Work out the finished part from the listing and answer in its coordinate system (mm). A direction names the side the tool comes from. Give positions to 0.01 mm unless a question says otherwise; leave off trailing zeros. Order: outer loops, then holes, each group sorted by start corner. A loop starts at its lowest first (then second) coordinate and runs counter-clockwise, first axis right, second up. Notation, with made-up numbers: (67.25, 52.5) -> (77.25, 52.5) arc R22 cw to (77.25, 80.5) -> close; hole circle Ø5 at (54.25, 74). An arc over 180 degrees is marked (long way). Use a Markdown table: item, result. Add a question column.
Autodesk Inventor part; units mm, degrees
ref_plane "YZ Plane" through (0, 0, 0) normal (1, 0, 0) x (0, 1, 0)
ref_plane "XZ Plane" through (0, 0, 0) normal (0, 1, 0) x (-1, 0, 0)
ref_plane "XY Plane" through (0, 0, 0) normal (0, 0, 1) x (1, 0, 0)
sketch "Sketch9" plane through (0, 0, 0) normal (0, 1, 0) x (-1, 0, 0)
  line L0 (15, 15) -> (-15, 15)
  line L1 (-15, 15) -> (-15, -15)
  line L2 (-15, -15) -> (15, -15)
  line L3 (15, -15) -> (15, 15)
  line L4 (15, 15) -> (-15, -15) construction
  line L5 (-15, 15) -> (15, -15) construction
  line L6 (-13, 13) -> (13, 13)
  line L7 (13, 13) -> (13, -13)
  line L8 (13, -13) -> (-13, -13)
  line L9 (-13, -13) -> (-13, 13)
  point P0 (0, 0)
  dimension "d172" = 30
  dimension "d173" = 30
  dimension "d174" = 2
extrude "Extrusion3" add sketch "Sketch9" against normal blind 345
sketch "Sketch10" plane through (0, 0, 0) normal (1, 0, 0) x (0, 1, 0)
  line L0 (0, 15) -> (0, -15) construction
  line L1 (0, 15) -> (-345, 15) construction
  line L2 (-345, -15) -> (-345, 15) construction
  line L3 (0, -15) -> (-345, -15) construction
  line L4 (-68.5, 8.5) -> (-51.5, 8.5)
  line L5 (-51.5, 8.5) -> (-51.5, -8.5)
  line L6 (-51.5, -8.5) -> (-68.5, -8.5)
  line L7 (-68.5, -8.5) -> (-68.5, 8.5)
  line L8 (-68.5, 8.5) -> (-51.5, -8.5) construction
  line L9 (-51.5, 8.5) -> (-68.5, -8.5) construction
  line L10 (0, 0) -> (30, 0)
  circle A0 centre (-60, 0) radius 8.5
  dimension "d177" = 17
  dimension "d178" = 17
  dimension "d181" = 30
  dimension "d182" = 90
extrude "Extrusion4" cut sketch "Sketch10" along normal through all contours A0
pattern_linear "Rectangular Pattern4" count 4 spacing 85 along (0, -1, 0) of "Extrusion4"
properties part number "SLM 1661 FDS 1000 way tube 1" material "Stainless Steel"
1) Straight lines are drawn through the part: line 1 (Y direction, x = 14.05, z = 0); line 2 (Z direction, x = 1.75, y = -172.5). For each, find the intervals that lie inside material, in ascending order.
2) The part is cut by section A-A, the plane x = 2.25. Determine the outline of the cut face in (y, z), then the cut area to 3 significant figures.
3) Which of the six approach directions +Z, -Z, +X, -X, +Y, -Y give full straight-line access (tool end or side, diameter ignored) to faces 1 (the cylindrical face through (13.99, -323.49, -0.37)), 2 (the flat face through (15, -170, 0)), 3 (the flat face through (-13, -170, 0))?
4) The part is cut by section B-B, the plane y = -162. Determine the outline of the cut face in (x, z).
5) Determine the mould class of faces 4 (the cylindrical face through (13.99, -136.89, -2.55)), 5 (the flat face through (13, -170, 0)), 6 (the cylindrical face through (13.99, -238.49, -0.37)), 7 (the flat face through (14, 0, 0)) for opening direction Y: released by +Y, released by -Y, zero draft, split by the parting line, or undercut.
6) The part is cut by section D-D, the plane y = -230. Determine the outline of the cut face in (x, z).
7) A flat-ended cylindrical pin translates along its axis: pin 1 (10 mm diameter, centred on y = -60, z = 0, fed in from +X). Find the tip coordinate at first contact, or state that the pin passes through.
8) The part is cut by section C-C, the plane z = 0. Determine the outline of the cut face in (x, y).
A:
| question | item | result |
|---|---|---|
| 1 | line 1 | -345 to -323.5, -306.5 to -238.5, -221.5 to -153.5, -136.5 to -68.5, -51.5 to 0 |
| 1 | line 2 | -15 to -13, 13 to 15 |
| 2 | outline | (-345, -15) -> (0, -15) -> (0, -13) -> (-345, -13) -> close; (-345, 13) -> (0, 13) -> (0, 15) -> (-345, 15) -> close |
| 2 | area | 1,380 mm^2 |
| 3 | face 1 | +X |
| 3 | face 2 | +Z, -Z, +X, +Y, -Y |
| 3 | face 3 | +Y, -Y |
| 4 | outline | (-15, -15) -> (15, -15) -> (15, 15) -> (-15, 15) -> close; hole (-13, -13) -> (13, -13) -> (13, 13) -> (-13, 13) -> close |
| 5 | face 4 | undercut |
| 5 | face 5 | zero draft |
| 5 | face 6 | undercut |
| 5 | face 7 | released by +Y |
| 6 | outline | (-15, -15) -> (15, -15) -> (15, -8.5) -> (13, -8.5) -> (13, -13) -> (-13, -13) -> (-13, 13) -> (13, 13) -> (13, 8.5) -> (15, 8.5) -> (15, 15) -> (-15, 15) -> close |
| 7 | pin 1 | x = -13 |
| 8 | outline | (-15, -345) -> (-13, -345) -> (-13, 0) -> (-15, 0) -> close; (13, -345) -> (15, -345) -> (15, -323.5) -> (13, -323.5) -> close; (13, -306.5) -> (15, -306.5) -> (15, -238.5) -> (13, -238.5) -> close; (13, -221.5) -> (15, -221.5) -> (15, -153.5) -> (13, -153.5) -> close; (13, -136.5) -> (15, -136.5) -> (15, -68.5) -> (13, -68.5) -> close; (13, -51.5) -> (15, -51.5) -> (15, 0) -> (13, 0) -> close |
